Geometry: see drawing. Coordinates: mm, zero at the bounding-box minimum. A direction names the side the tool comes from. Round coordinates to 2 decimals unless told otherwise and drop trailing zeros. Write each loop counter-clockwise with the first axis right and the second up, starting at its lowest first coordinate (ties: lowest second). Pieces come first, ordered by that corner, then holes. Notation, with made-up numbers: (11.5, -11) -> (17.5, -11) arc R10 ccw to (17.5, -6) -> close; hole circle Ø6 at (80, -12.5). An arc over 180 degrees is marked (long way). Use CSV: the item, a comma, the result in double quotes.
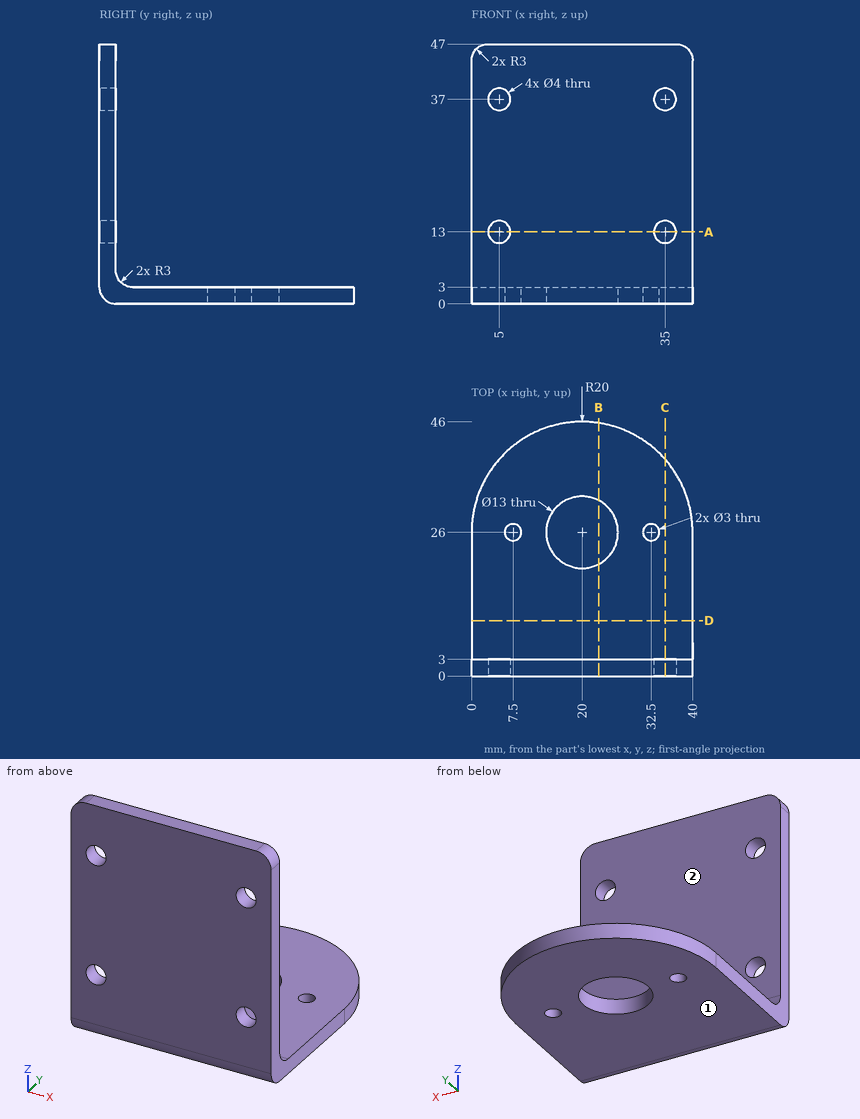
Item 1: First-contact query: pin 1 Ø1 at (x, z) = (24.5, 11) entering from +Y; pin 2 Ø5 at (x, y) = (7.5, 26) entering from +Z. Flat tips, straight axial feed; report the tip coordinate or a pass-through.
Worked answers:
pin 1,"stops at y = 3"
pin 2,"stops at z = 3"
Item 2: Section query A-A on z = 13. Return the cut outline in (x, y).
Worked answers:
outline,"(0, 0) -> (3, 0) -> (3, 3) -> (0, 3) -> close; (7, 0) -> (33, 0) -> (33, 3) -> (7, 3) -> close; (37, 0) -> (40, 0) -> (40, 3) -> (37, 3) -> close"
Item 3: Line query: line 1 (X direction, y = 1, z = 37); line 2 (Y direction, x = 20, z = 41). Output: solid intervals per line, ascending.
Worked answers:
line 1,"x = 0 to 3, 7 to 33, 37 to 40"
line 2,"y = 0 to 3"
Item 4: Section query B-B on x = 23. Return the cut outline in (y, z), plus the area to 3 significant figures.
Worked answers:
outline,"(0, 3) arc R3 ccw to (3, 0) -> (20.23, 0) -> (20.23, 3) -> (6, 3) arc R3 cw to (3, 6) -> (3, 47) -> (0, 47) -> close; (31.77, 0) -> (45.77, 0) -> (45.77, 3) -> (31.77, 3) -> close"
area,"235 mm²"
Item 5: Set-up query: the marked faces 1 and 2. Return all of +Z, -Z, +X, -X, +Y, -Y with unobstructed straight access to the full face (end or side cutting, diameter ignored); none if empty.
Worked answers:
face 1,"-Z, +X, -X, +Y, -Y"
face 2,"+Z, +X, -X, +Y"
Item 6: Section query D-D on y = 10. Return the cut outline in (x, z), plus the area to 3 significant figures.
Worked answers:
outline,"(0, 0) -> (40, 0) -> (40, 3) -> (0, 3) -> close"
area,"120 mm²"
Item 7: Section query C-C on x = 35. Return the cut outline in (y, z), plus the area to 3 significant figures.
Worked answers:
outline,"(0, 3) arc R3 ccw to (3, 0) -> (39.23, 0) -> (39.23, 3) -> (6, 3) arc R3 cw to (3, 6) -> (3, 11) -> (0, 11) -> close; (0, 15) -> (3, 15) -> (3, 35) -> (0, 35) -> close; (0, 39) -> (3, 39) -> (3, 47) -> (0, 47) -> close"
area,"226 mm²"
